```python
from build123d import *

# Parameters (mm, degrees)
F0_W     = 90
F0_H     = 110
F1_DEPTH = 3
F2_R     = 4
F2_R_2   = 1.5
F3_DEPTH = 10
F4_W     = 40
F4_H     = 110
F4_W_2   = 10
F4_H_2   = 12
F5_DEPTH = 2


with BuildPart() as f1:
    # F0 (on Front) → F1 (new body)
    with BuildSketch(Plane.XZ):
        Rectangle(F0_W, F0_H)
    extrude(amount=-F1_DEPTH)

    # F2 (on face) → F3 (join)
    with BuildSketch(Plane.XZ):
        with Locations((40, 50)):
            Circle(F2_R)
        with Locations((40, 50)):
            Circle(F2_R_2, mode=Mode.SUBTRACT)
        with Locations((-40, 50)):
            Circle(F2_R)
        with Locations((-40, 50)):
            Circle(F2_R_2, mode=Mode.SUBTRACT)
        with Locations((-40, -50)):
            Circle(F2_R)
        with Locations((-40, -50)):
            Circle(F2_R_2, mode=Mode.SUBTRACT)
        with Locations((40, -50)):
            Circle(F2_R)
        with Locations((40, -50)):
            Circle(F2_R_2, mode=Mode.SUBTRACT)
    extrude(amount=F3_DEPTH)

    # F4 (on face) → F5 (join)
    with BuildSketch(Plane(origin=(-45, 0, 0), x_dir=(0, -1, 0), z_dir=(-1, 0, 0))):
        with Locations((17, 0)):
            Rectangle(F4_W, F4_H)
        with Locations((18, 29)):
            Rectangle(F4_W_2, F4_H_2, mode=Mode.SUBTRACT)
    extrude(amount=F5_DEPTH)


solid = f1.part
```
The listing builds one solid part. Answer for the finished solid, in the listing's coordinates (mm). A direction names the side the tool comes from. Round coordinates to 2 decimals unless told otherwise and drop trailing zeros. Loops run counter-clockwise (first coordinate to the right, second up) from the corner with the lowest first, then second, coordinate; pieces in that order, holes last. Notation, with made-up numbers: (16.25, 24) - (72.25, 24) arc R13 ccw to (72.25, 41) - close; hole circle Ø8 at (-27.5, 45.5). An arc over 180 degrees is marked (long way). Return JSON: item names as keys, results as strings. Group by question number.
1. Consider probe 1 along Z at (x, y) = (40, -7); probe 2 along Y at (x, z) = (-17.5, -35); probe 3 along X at (y, z) = (-19.5, 2.5). Determine where each line is inside the solid, lowest interval first.
2. Each of these flat-tipped pins is pushed along its axis until it touches: P1, Ø1.5, axis at x = 40.5, z = -50, coming from the -Y side; P2, Ø2.5, axis at x = -38, z = 50, coming from the -Y side; P3, Ø4, axis at y = -31.5, z = -4.5, coming from the +X side. Where does it stop, or does it pass through?
3. Which of the six approach directions +Z, -Z, +X, -X, +Y, -Y give full straight-line access (tool end or side, diameter ignored) to faces 4 (the flat face through (40, -10, 48)), 5 (the flat face through (-47, -17, 1)), 6 (the cylindrical face through (-41.2, -4.9, 49.1))?
4. The part is cut by section A-A on y = -7. State how many separate pieces and enclosed holes the cut face has, then the cut area to 3 significant figures.
5. The part is cut by section C-C on x = 40. Determine the outline of the cut face in (y, z), then the cut area to 3 significant figures.
6. The part is cut by section D-D on z = 20. Determine the outline of the cut face in (x, y).
7. The part is cut by section B-B on z = 50. Determine the outline of the cut face in (x, y).
8. The mould has two halves that part along Z. Classify faces 1 (the flat face through (-14, 1, 55)), 2 (the flat face through (-45, -18, 1)), 3 (the flat face through (-40, 0, 50)): pulls with the +Z half, pulls with the -Z half, needs draft (parallel to the pull), parting line crosses it, or undercut.
Resolved:
{
 "1": {"probe 1": "z = -54 to -51.5, -48.5 to -46, 46 to 48.5, 51.5 to 54", "probe 2": "y = 0 to 3", "probe 3": "x = -47 to -45"},
 "2": {"P1": "stops at y = 0", "P2": "stops at y = -10", "P3": "stops at x = -45"},
 "3": {"face 4": "+Z, -Z, +X, -Y", "face 5": "+Z, -Z, -X, +Y, -Y", "face 6": "-Y"},
 "4": {"separate pieces": "5", "enclosed holes": "4", "area": "393 mm²"},
 "5": {"outline": "(-10, -54) - (0, -54) - (0, -55) - (3, -55) - (3, 55) - (0, 55) - (0, 54) - (-10, 54) - (-10, 51.5) - (0, 51.5) - (0, 48.5) - (-10, 48.5) - (-10, 46) - (0, 46) - (0, -46) - (-10, -46) - (-10, -48.5) - (0, -48.5) - (0, -51.5) - (-10, -51.5) - close", "area": "430 mm²"},
 "6": {"outline": "(-47, -37) - (-45, -37) - (-45, 0) - (45, 0) - (45, 3) - (-47, 3) - close"},
 "7": {"outline": "(-47, -37) - (-45, -37) - (-45, 0) - (-44, 0) - (-44, -10) - (-41.5, -10) - (-41.5, 0) - (-38.5, 0) - (-38.5, -10) - (-36, -10) - (-36, 0) - (36, 0) - (36, -10) - (38.5, -10) - (38.5, 0) - (41.5, 0) - (41.5, -10) - (44, -10) - (44, 0) - (45, 0) - (45, 3) - (-47, 3) - close"},
 "8": {"face 1": "pulls with the +Z half", "face 2": "needs draft", "face 3": "undercut"}
}
